```python
from build123d import *

# Parameters (mm, degrees)
SKETCH1_R           = 0.95
SKETCH1_R_2         = 0.7
BOSS_EXTRUDE1_DEPTH = 4
SKETCH2_W           = 16.2
SKETCH2_H           = 11.795
CUT_EXTRUDE1_DEPTH  = 2


with BuildPart() as part:
    # Sketch1 → Boss-Extrude1 (new body)
    with BuildSketch(Plane.XY):
        with BuildLine():
            Line((0, 6), (0, 11.795))
            ThreePointArc((0, 11.795), (1.464466094, 15.330533906), (5, 16.795))
            Line((5, 16.795), (11.2, 16.795))
            ThreePointArc((11.2, 16.795), (14.735533906, 15.330533906), (16.2, 11.795))
            Line((16.2, 11.795), (16.2, 6))
            Line((16.2, 6), (12.2, 6))
            Line((12.2, 6), (12.2, 4))
            Line((12.2, 4), (16.2, 4))
            Line((16.2, 4), (16.2, 2))
            ThreePointArc((16.2, 2), (15.614213562, 0.585786438), (14.2, 0))
            Line((14.2, 0), (2, 0))
            ThreePointArc((2, 0), (0.585786438, 0.585786438), (0, 2))
            Line((0, 2), (0, 4))
            Line((0, 4), (4, 4))
            Line((4, 4), (4, 6))
            Line((4, 6), (0, 6))
        make_face()
        with Locations((13.25, 2)):
            Circle(SKETCH1_R, mode=Mode.SUBTRACT)
        with Locations((13.25, 8)):
            Circle(SKETCH1_R, mode=Mode.SUBTRACT)
        with Locations((3, 13.795)):
            Circle(SKETCH1_R_2, mode=Mode.SUBTRACT)
        with Locations((13.2, 13.795)):
            Circle(SKETCH1_R_2, mode=Mode.SUBTRACT)
        with Locations((2.95, 8)):
            Circle(SKETCH1_R, mode=Mode.SUBTRACT)
        with Locations((2.95, 2)):
            Circle(SKETCH1_R, mode=Mode.SUBTRACT)
    extrude(amount=BOSS_EXTRUDE1_DEPTH)

    # Sketch2 → Cut-Extrude1 (cut)
    with BuildSketch(Plane.XY):
        with Locations((8.1, 5.8975)):
            Rectangle(SKETCH2_W, SKETCH2_H)
    extrude(amount=CUT_EXTRUDE1_DEPTH, mode=Mode.SUBTRACT)


solid = part.part
```
Can you work these out from the model? Positions are in its coordinate system, mm. A direction names the side the tool comes from. Give positions to 0.01 mm unless a question says otherwise; leave off trailing zeros. Loops run counter-clockwise (first coordinate to the right, second up) from the corner with the lowest first, then second, coordinate; pieces in that order, holes last. Notation, with made-up numbers: M -40,-11.5 L -25,-11.5 A33 ccw -25,20.5 Z; hole C 48,46 d4. An arc over 180 degrees is marked long. Use one line per item in the form item = value. Start each with the question number.
(1) I want a section at A-A, the plane y = 8. Write out the boundary of the cut face in (x, z), and give its area (3 significant figures).
(2) On a 3-axis mill with a long thin cutter (end or side, diameter ignored), from which of +Z, -Z, +X, -X, +Y, -Y can I reach the whole of each face in a straight line? I mean faces 5 (the flat face through (4, 5, 3)), 6 (the flat face through (14, 4, 3)), 7 (the cylindrical face through (15.63, 0.6, 2.99)). Say none if no direction works.
(3) I want a section at B-B, the plane x = 3. Write out the boundary of the cut face in (y, z) (3 decimals).
(4) I want a section at D-D, the plane z = 2.45. Write out the boundary of the cut face in (x, y) (3 decimals), and give its area (3 significant figures).
(5) Thinking about a two-plate mould opening in Y: for faces 1 (the cylindrical face through (14.156, 2.285, 2.986)), 2 (the flat face through (8, 11.795, 1)), 3 (the flat face through (2, 4, 3)), 4 (the flat face through (0, 9, 3)), which applies, released by +Y, released by -Y, zero draft, split by the parting line, or undercut?
(6) I'm going to push flat-ended pins straight in: P1, Ø1.1, axis at x = 2.95, y = 8, coming from the -Z side (3 decimals); P2, Ø2, axis at x = 13.5, z = 1.5, coming from the +Y side; P3, Ø0.6, axis at x = 14, z = 3, coming from the +Y side; P4, Ø0.6, axis at x = 2.5, z = 2.5, coming from the +Y side (3 decimals). Where does each tip first touch, or does it pass through?
(7) Please list where these lines run through material, in increasing order: line 1 (X direction, y = 2, z = 3.3); line 2 (X direction, y = 8.75, z = 2.05); line 3 (Y direction, x = 2.95, z = 3.35).
(8) I want a section at C-C, the plane z = 0.75. Write out the boundary of the cut face in (x, y) (3 decimals), and give its area (3 significant figures).
Worked out:
q1.outline = M 0,2 L 2,2 L 2,4 L 0,4 Z; M 3.9,2 L 12.3,2 L 12.3,4 L 3.9,4 Z; M 14.2,2 L 16.2,2 L 16.2,4 L 14.2,4 Z
q1.area = 24.8 mm²
q2.face_5 = +Z, -Z, -X
q2.face_6 = +Z, -Z, +X
q2.face_7 = +Z, -Z, +X, -Y
q3.outline = M 0,2 L 1.051,2 L 1.051,4 L 0,4 Z; M 2.949,2 L 4,2 L 4,4 L 2.949,4 Z; M 6,2 L 7.051,2 L 7.051,4 L 6,4 Z; M 8.949,2 L 11.795,2 L 11.795,0 L 13.095,0 L 13.095,4 L 8.949,4 Z; M 14.495,0 L 16.378,0 L 16.378,4 L 14.495,4 Z
q4.outline = M 0,2 A2 ccw 2,0 L 14.2,0 A2 ccw 16.2,2 L 16.2,4 L 12.2,4 L 12.2,6 L 16.2,6 L 16.2,11.795 A5 ccw 11.2,16.795 L 5,16.795 A5 ccw 0,11.795 L 0,6 L 4,6 L 4,4 L 0,4 Z; hole C 2.95,2 d1.9; hole C 2.95,8 d1.9; hole C 3,13.795 d1.4; hole C 13.25,2 d1.9; hole C 13.25,8 d1.9; hole C 13.2,13.795 d1.4
q4.area = 229 mm²
q5.face_1 = undercut
q5.face_2 = released by -Y
q5.face_3 = undercut
q5.face_4 = zero draft
q6.P1 = through
q6.P2 = 16.62
q6.P3 = 16.13
q6.P4 = 16.285
q7.line_1 = 0 to 2, 3.9 to 12.3, 14.2 to 16.2
q7.line_2 = 0 to 2.37, 3.53 to 12.67, 13.83 to 16.2
q7.line_3 = 0 to 1.05, 2.95 to 4, 6 to 7.05, 8.95 to 13.1, 14.49 to 16.36
q8.outline = M 0,11.795 L 16.2,11.795 A5 ccw 11.2,16.795 L 5,16.795 A5 ccw Z; hole C 3,13.795 d1.4; hole C 13.2,13.795 d1.4
q8.area = 67.2 mm²
